from build123d import *

# Parameters (mm, degrees)
SKETCH1_R           = 7.55
SKETCH1_R_2         = 6.05
BOSS_EXTRUDE1_DEPTH = 4
BOSS_EXTRUDE2_START = -4
SKETCH1_4_R         = 8.55
BOSS_EXTRUDE2_DEPTH = 2.5
SKETCH1_5_R         = 6.05
BOSS_EXTRUDE3_DEPTH = 17


with BuildPart() as part:
    # Sketch1 → Boss-Extrude1 (new body)
    # profile 1 of 2: a face of its own
    with BuildSketch(Plane(origin=(0, 0, 0), x_dir=(1, 0, 0), z_dir=(0, 1, 0))):
        with Locations(Location((-1.5, 0, 0), (0, 0, 270))):
            Circle(SKETCH1_R)
        Circle(SKETCH1_R_2, mode=Mode.SUBTRACT)
    # profile 2 of 2: a face of its own
    with BuildSketch(Plane(origin=(0, 0, 0), x_dir=(1, 0, 0), z_dir=(0, 1, 0))):
        Circle(SKETCH1_R_2)
        Polygon((2.886751346, -5), (5.773502692, 0), (2.886751346, 5), (-2.886751346, 5), (-5.773502692, 0), (-2.886751346, -5), align=None, mode=Mode.SUBTRACT)
    extrude(amount=-BOSS_EXTRUDE1_DEPTH)

    # Sketch1<4> → Boss-Extrude2 (add)
    with BuildSketch(Plane(origin=(0, 0, 0), x_dir=(1, 0, 0), z_dir=(0, 1, 0)).offset(BOSS_EXTRUDE2_START)):
        with Locations(Location((-1.5, 0, 0), (0, 0, 270))):
            Circle(SKETCH1_4_R)
        Polygon((5.773502692, 0), (2.886751346, 5), (-2.886751346, 5), (-5.773502692, 0), (-2.886751346, -5), (2.886751346, -5), align=None, mode=Mode.SUBTRACT)
    extrude(amount=-BOSS_EXTRUDE2_DEPTH)

    # Sketch1<5> → Boss-Extrude3 (add)
    with BuildSketch(Plane(origin=(0, 0, 0), x_dir=(1, 0, 0), z_dir=(0, 1, 0))):
        Circle(SKETCH1_5_R)
        Polygon((2.886751346, -5), (5.773502692, 0), (2.886751346, 5), (-2.886751346, 5), (-5.773502692, 0), (-2.886751346, -5), align=None, mode=Mode.SUBTRACT)
    extrude(amount=BOSS_EXTRUDE3_DEPTH)


solid = part.part
The listing builds one solid part. Answer for the finished solid, in the listing's coordinates (mm). A direction names the side the tool comes from. Round coordinates to 2 decimals unless told otherwise and drop trailing zeros. Order: outer loops, then holes, each group sorted by start corner. A loop starts at its lowest first (then second) coordinate and runs counter-clockwise, first axis right, second up. Notation, with made-up numbers: M 24,-28 L 40,-28 A26 ccw 40,-2 Z; hole C 13,47.25 d3. An arc over 180 degrees is marked long. Answer in a Markdown table with one row per item. Add a question column.
1) Which of the six approach directions +Z, -Z, +X, -X, +Y, -Y give full straight-line access (tool end or side, diameter ignored) to faces 4 (the face through (5.589, 8.381, 2.317)), 5 (the face through (4.35, 5.086, -2.465)), 6 (the face through (-5, -6.5, 2))?
2) Consider line 1 along Z through (x, y) = (0.25, 6); line 2 along Y through (x, z) = (-4.75, -6.25); line 3 along X through (y, z) = (14.25, 3.75). Determine where each line is inside the solid, lowest interval first. Write a range as from..to.
3) The part is cut by section D-D on x = -7. Determine the outline of the cut face in (y, z), plus the area to 3 significant figures.
4) The part is cut by section C-C on x = 0. Determine the outline of the cut face in (y, z).
5) The part is cut by section A-A on y = 14.5. Determine the outline of the cut face in (x, z).
6) Flat-ended cylindrical pins translate along their axes: pin 1 Ø3 at (y, z) = (-1, -4) entering from +X; pin 2 Ø8 at (x, y) = (-7.5, 5) entering from -Z; pin 3 Ø1.7 at (x, y) = (-0.5, 8.5) entering from +Z. Find the tip coordinate at first contact, or state that the pin passes through.
7) Determine the mould class of faces 1 (the face through (1.068, -5.232, 8.155)), 2 (the face through (-4.35, 5.086, 2.465)), 3 (the face through (-7, -4, 6)) for opening direction Z: pulls with the +Z half, pulls with the -Z half, needs draft (parallel to the pull), parting line crosses it, or undercut.
Findings below:
| question | item | result |
|---|---|---|
| 1 | face 4 | +Y |
| 1 | face 5 | +Y, -Y |
| 1 | face 6 | +Z, -Z, +X, -X, -Y |
| 2 | line 1 | z = -6.04..-5, 5..6.04 |
| 2 | line 2 | y = -6.5..0 |
| 2 | line 3 | x = -4.75..-3.61, 3.61..4.75 |
| 3 | outline | M -6.5,-6.55 L -4,-6.55 L -4,-5.17 L 0,-5.17 L 0,5.17 L -4,5.17 L -4,6.55 L -6.5,6.55 Z |
| 3 | area | 74.1 mm² |
| 4 | outline | M -6.5,-8.42 L -4,-8.42 L -4,-7.4 L 0,-7.4 L 0,-6.05 L 17,-6.05 L 17,-5 L -6.5,-5 Z; M -6.5,5 L 17,5 L 17,6.05 L 0,6.05 L 0,7.4 L -4,7.4 L -4,8.42 L -6.5,8.42 Z |
| 5 | outline | C 0,0 d12.1; hole M -5.77,0 L -2.89,-5 L 2.89,-5 L 5.77,0 L 2.89,5 L -2.89,5 Z |
| 6 | pin 1 | stops at x = 5.62 |
| 6 | pin 2 | stops at z = -4.93 |
| 6 | pin 3 | stops at z = 6.05 |
| 7 | face 1 | parting line crosses it |
| 7 | face 2 | undercut |
| 7 | face 3 | needs draft |
